Verification items for the finished model (mm, model axes). A direction names the side the tool comes from. Coordinates: 2 decimals unless noted, no trailing zeros. Loops run counter-clockwise (first coordinate to the right, second up) from the corner with the lowest first, then second, coordinate; pieces in that order, holes last. Notation, with made-up numbers: (-37, -4) - (1, -4) arc R21 ccw to (1, 21) - close; hole circle Ø6 at (35, 22.25). An arc over 180 degrees is marked (long way). Answer as CSV lines item,"result". Start each with the question number.
1. Material ranges on line 1 (X direction, y = 5.25, z = -50.5) (3 decimals); line 2 (X direction, y = 11.25, z = -5); line 3 (Z direction, x = 8, y = 10.5), recorded low to high. Write a range as [from, to].
2. Set-up check for faces 4 (the cylindrical face through (18.27, 7.94, -4.46)), 5 (the flat face through (8, 9, -17.314)): record each of +Z, -Z, +X, -X, +Y, -Y from which the full face is reachable in a straight line by a thin tool's end or side.
3. Cross-section at B-B (x = -8.5). Enter the section's corners in (y, z), plus the area to 3 significant figures.
4. Release check for a two-part mould opening along Z. For faces 1 (the flat face through (39.56, 9, -37)), 2 (the flat face through (-1, 6, -68.162)), 3 (the flat face through (-32, 12.7, -31)) record: pulls with the +Z half, pulls with the -Z half, needs draft (parallel to the pull), parting line crosses it, or undercut.
5. Gauge pin test, flat end, axial feed: P1, Ø10, axis at x = -4, z = -23.5, coming from the +Y side. Record the tip position at first contact, or that the pin passes through.
6. Cross-section at A-A (z = -20). Enter the section's corners in (x, y) (3 decimals), plus the area to 3 significant figures.
```python
from build123d import *

# Parameters (mm, degrees)
SKETCH1_W           = 101.6
SKETCH1_H           = 76.2
BOSS_EXTRUDE1_DEPTH = 12.7
SKETCH4_W           = 62.685063192
SKETCH4_H           = 39.138657103
CUT_EXTRUDE2_DEPTH  = 7.62
SKETCH5_R           = 3.175
SKETCH5_R_2         = 4.7625
CUT_EXTRUDE3_DEPTH  = 93.457395594


with BuildPart() as part:
    # Sketch1 → Boss-Extrude1 (new body)
    with BuildSketch(Plane(origin=(0, 0, 0), x_dir=(1, 0, 0), z_dir=(0, 1, 0))):
        with Locations((0, 30.062025316)):
            Rectangle(SKETCH1_W, SKETCH1_H)
    extrude(amount=BOSS_EXTRUDE1_DEPTH)

    # Sketch4 → Cut-Extrude2 (cut)
    with BuildSketch(Plane(origin=(0, 12.7, 0), x_dir=(1, 0, 0), z_dir=(0, 1, 0))):
        with Locations((8.217537696, 36.883635135)):
            Rectangle(SKETCH4_W, SKETCH4_H)
    extrude(amount=-CUT_EXTRUDE2_DEPTH, mode=Mode.SUBTRACT)

    # Sketch5 → Cut-Extrude3 (cut, through all)
    with BuildSketch(Plane.XY.offset(8.037974684)):
        with Locations((0.917080185, 12.7)):
            Circle(SKETCH5_R)
        with Locations((18.379580185, 12.7)):
            Circle(SKETCH5_R_2)
    extrude(amount=-CUT_EXTRUDE3_DEPTH, mode=Mode.SUBTRACT)


solid = part.part
```
Values follow:
1,line 1,"x = [-50.8, -23.125], [39.56, 50.8]"
1,line 2,"x = [-50.8, -1.91], [3.74, 13.84], [22.92, 50.8]"
1,line 3,"z = [-68.16, -56.45], [-17.31, 8.04]"
2,face 4,"+Z, -Z, +Y"
2,face 5,"+Y"
3,outline,"(0, -68.16) - (12.7, -68.16) - (12.7, -56.45) - (5.08, -56.45) - (5.08, -17.31) - (12.7, -17.31) - (12.7, 8.04) - (0, 8.04) - close"
3,area,"670 mm²"
4,face 1,"undercut"
4,face 2,"pulls with the -Z half"
4,face 3,"needs draft"
5,P1,"stops at y = 5.08"
6,outline,"(-50.8, 0) - (50.8, 0) - (50.8, 12.7) - (39.56, 12.7) - (39.56, 5.08) - (-23.125, 5.08) - (-23.125, 12.7) - (-50.8, 12.7) - close"
6,area,"813 mm²"
